Design review of the part shown in the three views and the two pictorial views. Dimensions are in mm from the part's minimum x, y and z. Round coordinates to 2 decimals unless told otherwise and drop trailing zeros. Loops run counter-clockwise (first coordinate to the right, second up) from the corner with the lowest first, then second, coordinate; pieces in that order, holes last.
1) Wall thickness on L1, parallel to X at y = 90, z = 2.8 (3 decimals); L2, parallel to Y at x = 7, z = 4: over which ranges is each line inside the solid? List them lowest first.
2) Insertion check: pin 1 (2.5 mm diameter, centred on x = 68.105, y = 90, fed in from -Z). The pin has a flat end and moves straight along its axis. Give the tip position at first contact, or say it passes through.
3) Take a section at B-B (z = 4). Give the number of separate pieces and of enclosed holes in the cut face, then the cut area to 3 significant figures.
4) Take a section at A-A (y = 10). State the section outline as (x, z) points (3 decimals).
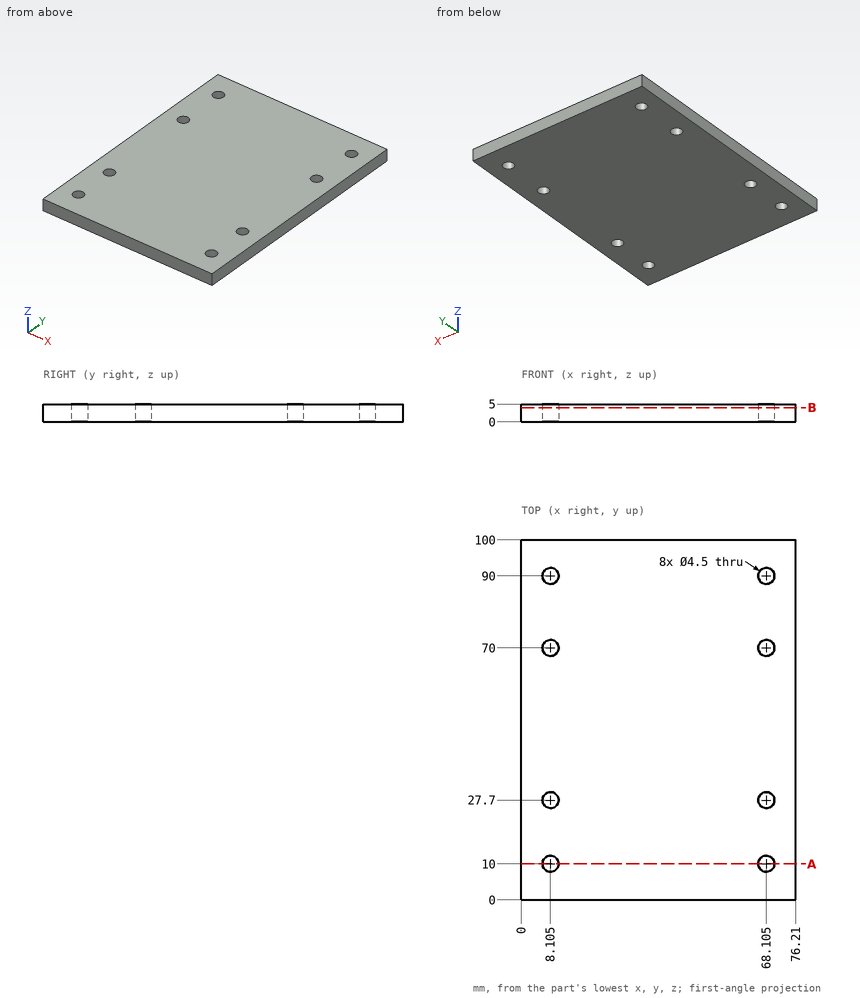
Response:
1. L1: x = 0 to 5.855, 10.355 to 65.855, 70.355 to 76.21
1. L2: y = 0 to 8.04, 11.96 to 25.74, 29.66 to 68.04, 71.96 to 88.04, 91.96 to 100
2. pin 1: passes through
3. separate pieces: 1
3. enclosed holes: 8
3. area: 7,490 mm2
4. outline: (0, 0) - (5.855, 0) - (5.855, 5) - (0, 5) - close; (10.355, 0) - (65.855, 0) - (65.855, 5) - (10.355, 5) - close; (70.355, 0) - (76.21, 0) - (76.21, 5) - (70.355, 5) - close
